from build123d import *

# Parameters (mm, degrees)
SKETCH1_R             = 9.5
BOSS_EXTRUDE1_DEPTH   = 22.5
M4_TAPPED_HOLE1_D     = 3.3
M4_TAPPED_HOLE1_DEPTH = 10.1
M4_TAPPED_HOLE1_TIP   = 0.991420021
M4_TAPPED_HOLE2_D     = 3.3
M4_TAPPED_HOLE2_DEPTH = 15
M4_TAPPED_HOLE2_TIP   = 0.991420021


with BuildPart() as part:
    # Sketch1 → Boss-Extrude1 (new, symmetric)
    # profile 1 of 2: a face of its own
    with BuildSketch(Plane.XY):
        with BuildLine():
            Line((-55, 0), (0, 0))
            Line((0, 0), (0, 5))
            ThreePointArc((0, 5), (-15, 20), (0, 35))
            Line((0, 35), (0, 40))
            Line((0, 40), (-45, 40))
            Line((-45, 40), (-55, 40))
            Line((-55, 40), (-55, 0))
        make_face()
        with Locations(Location((-30, 20, 0), (0, 0, 180))):
            Circle(SKETCH1_R, mode=Mode.SUBTRACT)
    # profile 2 of 2: a face of its own
    with BuildSketch(Plane.XY):
        with BuildLine():
            Line((0, 5), (0, 0))
            Line((0, 0), (55, 0))
            Line((55, 0), (55, 40))
            Line((55, 40), (45, 40))
            Line((45, 40), (0, 40))
            Line((0, 40), (0, 35))
            ThreePointArc((0, 35), (10.606601718, 30.606601718), (15, 20))
            ThreePointArc((15, 20), (10.606601718, 9.393398282), (0, 5))
        make_face()
        with Locations(Location((30, 20, 0), (0, 0, 180))):
            Circle(SKETCH1_R, mode=Mode.SUBTRACT)
    extrude(amount=BOSS_EXTRUDE1_DEPTH, both=True)

    # M4 Tapped Hole1
    with Locations(Plane(origin=(0, 0, -22.5), x_dir=(-1, 0, 0), z_dir=(0, 0, -1))):
        with Locations((12, 32), (-12, 32), (12, 8), (-12, 8)):
            Hole(M4_TAPPED_HOLE1_D / 2, depth=M4_TAPPED_HOLE1_DEPTH)
            with Locations((0, 0, -(M4_TAPPED_HOLE1_DEPTH + M4_TAPPED_HOLE1_TIP / 2))):  # 118° drill point
                Cone(0, M4_TAPPED_HOLE1_D / 2, M4_TAPPED_HOLE1_TIP, mode=Mode.SUBTRACT)

    # M4 Tapped Hole2
    with Locations(Plane(origin=(0, 40, 0), x_dir=(1, 0, 0), z_dir=(0, 1, 0))):
        with Locations((47, 14.5), (-47, 14.5), (-47, -14.5), (47, -14.5)):
            Hole(M4_TAPPED_HOLE2_D / 2, depth=M4_TAPPED_HOLE2_DEPTH)
            with Locations((0, 0, -(M4_TAPPED_HOLE2_DEPTH + M4_TAPPED_HOLE2_TIP / 2))):  # 118° drill point
                Cone(0, M4_TAPPED_HOLE2_D / 2, M4_TAPPED_HOLE2_TIP, mode=Mode.SUBTRACT)


solid = part.part
Geometry: final body of the model. Coordinates: model frame, mm. A direction names the side the tool comes from. Round coordinates to 2 decimals unless told otherwise and drop trailing zeros. Write each loop counter-clockwise with the first axis right and the second up, starting at its lowest first coordinate (ties: lowest second). Pieces come first, ordered by that corner, then holes. Notation, with made-up numbers: M 70.25,42 L 122.25,42 A16 cw 122.25,62 Z; hole C 76.5,-22 d3. An arc over 180 degrees is marked long. Write item = value, one per line.
Item 1: Access query for faces 1 (the face through (-45.35, 32.39, -14.57)), 2 (the face through (13.574, 8.496, -17.379)). Directions: +Z, -Z, +X, -X, +Y, -Y. A direction counts if a zero-diameter tool reaches every point of the face in a straight line with its end or side. Return the directions, or none.
Findings:
face_1 = +Y
face_2 = -Z
Item 2: Material intervals for line 1 along X through (y, z) = (26.5, 3.5); line 2 along X through (y, z) = (8, -14); line 3 along X through (y, z) = (32, -16), sorted ascending. Write a range as [from, to].
Findings:
line_1 = [-55, -36.93], [-23.07, -13.52], [13.52, 23.07], [36.93, 55]
line_2 = [-55, -13.65], [-10.35, -9], [9, 10.35], [13.65, 55]
line_3 = [-55, -47.69], [-46.31, -13.65], [-10.35, -9], [9, 10.35], [13.65, 46.31], [47.69, 55]
Item 3: Section query B-B on z = 10. Return loops of the section in (x, y), then the cut area to 3 significant figures.
Findings:
outline = M -55,0 L 55,0 L 55,40 L -55,40 Z; hole C -30,20 d19; hole C 0,20 d30; hole C 30,20 d19
area = 3,130 mm^2
Item 4: Section query C-C on x = -34. Return loops of the section in (y, z), then the cut area to 3 significant figures.
Findings:
outline = M 0,-22.5 L 11.38,-22.5 L 11.38,22.5 L 0,22.5 Z; M 28.62,-22.5 L 40,-22.5 L 40,22.5 L 28.62,22.5 Z
area = 1,020 mm^2
Item 5: Section query A-A on x = 30. Return loops of the section in (y, z).
Findings:
outline = M 0,-22.5 L 10.5,-22.5 L 10.5,22.5 L 0,22.5 Z; M 29.5,-22.5 L 40,-22.5 L 40,22.5 L 29.5,22.5 Z
Item 6: Pin query (flat end, axial travel): P1, Ø2, axis at x = 12, y = 32, coming from the -Z side; P2, Ø5.5, axis at x = 12, y = 8, coming from the -Z side; P3, Ø2, axis at x = -47, z = 14.5, coming from the +Y side. Return the tip coordinate at first contact, or that it passes through.
Findings:
P1 = -12.01
P2 = -22.5
P3 = 24.61
Item 7: Pull-direction query (Y, two-part tool) for faces 3 (the face through (-45.35, 32.39, 14.43)), 4 (the face through (12.23, 31.83, -11.58)), 5 (the face through (-47.21, 24.18, 14.31)); classes: pulls with the +Y half, pulls with the -Y half, needs draft (parallel to the pull), parting line crosses it, or undercut.
Findings:
face_3 = needs draft
face_4 = undercut
face_5 = pulls with the +Y half
